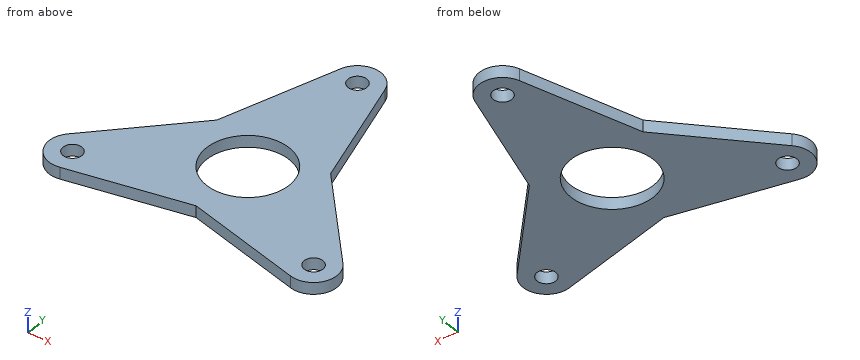
```python
from build123d import *

# Parameters (mm, degrees)
SKETCH3_R           = 11.176
SKETCH3_R_2         = 2.54
BOSS_EXTRUDE2_DEPTH = 3.175


with BuildPart() as part:
    # Sketch3 → Boss-Extrude2 (new body)
    with BuildSketch(Plane.XY):
        with BuildLine():
            Line((-6.070664946, 39.962666667), (-15.573595811, 8.991419734))
            Line((-15.573595811, 8.991419734), (-37.644017009, -14.723983272))
            ThreePointArc((-37.644017009, -14.723983272), (-38.494829198, -22.225), (-31.573352063, -25.238683395))
            Line((-31.573352063, -25.238683395), (0, -17.982839467))
            Line((0, -17.982839467), (31.573352063, -25.238683395))
            ThreePointArc((31.573352063, -25.238683395), (38.494829198, -22.225), (37.644017009, -14.723983272))
            Line((37.644017009, -14.723983272), (15.573595811, 8.991419734))
            Line((15.573595811, 8.991419734), (6.070664946, 39.962666667))
            ThreePointArc((6.070664946, 39.962666667), (0, 44.45), (-6.070664946, 39.962666667))
        make_face()
        Circle(SKETCH3_R, mode=Mode.SUBTRACT)
        with Locations((0, 38.1)):
            Circle(SKETCH3_R_2, mode=Mode.SUBTRACT)
        with Locations((32.995567884, -19.05)):
            Circle(SKETCH3_R_2, mode=Mode.SUBTRACT)
        with Locations((-32.995567884, -19.05)):
            Circle(SKETCH3_R_2, mode=Mode.SUBTRACT)
    extrude(amount=BOSS_EXTRUDE2_DEPTH)


solid = part.part
```
Geometry: final body of the model. Coordinates: model frame, mm. Round coordinates to 2 decimals unless told otherwise and drop trailing zeros. Order: outer loops, then holes, each group sorted by start corner. A loop starts at its lowest first (then second) coordinate and runs counter-clockwise, first axis right, second up. Notation, with made-up numbers: (57.5, -35.75) - (100.5, -35.75) arc R20 cw to (100.5, 2.25) - close; hole circle Ø8 at (19.5, -40). An arc over 180 degrees is marked (long way). Write item = value, one per line. Start each with the question number.
Q1. Cut plane D-D on y = 38.1. Return the cut outline in (x, z) (3 decimals), and give its area (3 significant figures).
Q2. Cut plane C-C on y = -20. Return the cut outline in (x, z) (3 decimals).
Q3. Ray query, line 1 (Y direction, x = 0, z = 1); line 2 (Y direction, x = 1, z = 1.75); line 3 (X direction, y = -5.5, z = 2.1). Return the intervals inside material, ascending. Write a range as from..to.
Q4. Cut plane B-B on z = 0.8. Return the cut outline in (x, y), and give its area (3 significant figures).
Q5. Cut plane A-A on y = -2. Return the cut outline in (x, z) (3 decimals), and give its area (3 significant figures).
Outcome:
q1.outline = (-6.642, 0) - (-2.54, 0) - (-2.54, 3.175) - (-6.642, 3.175) - close; (2.54, 0) - (6.642, 0) - (6.642, 3.175) - (2.54, 3.175) - close
q1.area = 26.0 mm^2
q2.outline = (-39.274, 0) - (-35.351, 0) - (-35.351, 3.175) - (-39.274, 3.175) - close; (-30.64, 0) - (-8.778, 0) - (-8.778, 3.175) - (-30.64, 3.175) - close; (8.778, 0) - (30.64, 0) - (30.64, 3.175) - (8.778, 3.175) - close; (35.351, 0) - (39.274, 0) - (39.274, 3.175) - (35.351, 3.175) - close
q3.line_1 = -17.98..-11.18, 11.18..35.56, 40.64..44.45
q3.line_2 = -18.21..-11.13, 11.13..35.77, 40.43..44.37
q3.line_3 = -29.06..-9.73, 9.73..29.06
q4.outline = (-37.64, -14.72) arc R6.35 ccw to (-31.57, -25.24) - (0, -17.98) - (31.57, -25.24) arc R6.35 ccw to (37.64, -14.72) - (15.57, 8.99) - (6.07, 39.96) arc R6.35 ccw to (-6.07, 39.96) - (-15.57, 8.99) - close; hole circle Ø5.08 at (-33, -19.05); hole circle Ø22.35 at (0, 0); hole circle Ø5.08 at (0, 38.1); hole circle Ø5.08 at (33, -19.05)
q4.area = 2,100 mm^2
q5.outline = (-25.803, 0) - (-10.996, 0) - (-10.996, 3.175) - (-25.803, 3.175) - close; (10.996, 0) - (25.803, 0) - (25.803, 3.175) - (10.996, 3.175) - close
q5.area = 94.0 mm^2
